from build123d import *

# Parameters (mm, degrees)
F0_R     = 25
F0_R_2   = 1.25
F1_DEPTH = 3


with BuildPart() as f1:
    # F0 (on Top) → F1 (new body)
    with BuildSketch(Plane.XY):
        Circle(F0_R)
        with BuildLine():
            Line((-2, -21.25), (-2, -19.25))
            ThreePointArc((-2, -19.25), (0, -17.25), (2, -19.25))
            Line((2, -19.25), (2, -21.25))
            ThreePointArc((2, -21.25), (0, -23.25), (-2, -21.25))
        make_face(mode=Mode.SUBTRACT)
        with Locations((0, -11.25)):
            Circle(F0_R_2, mode=Mode.SUBTRACT)
        with BuildLine():
            Line((-19.25, -2), (-21.25, -2))
            ThreePointArc((-21.25, -2), (-23.25, 0), (-21.25, 2))
            Line((-21.25, 2), (-19.25, 2))
            ThreePointArc((-19.25, 2), (-17.25, 0), (-19.25, -2))
        make_face(mode=Mode.SUBTRACT)
        with Locations((-11.25, 0)):
            Circle(F0_R_2, mode=Mode.SUBTRACT)
        with Locations((11.25, 0)):
            Circle(F0_R_2, mode=Mode.SUBTRACT)
        with Locations((0, 11.25)):
            Circle(F0_R_2, mode=Mode.SUBTRACT)
        with BuildLine():
            ThreePointArc((21.25, 2), (23.25, 0), (21.25, -2))
            Line((21.25, -2), (19.25, -2))
            ThreePointArc((19.25, -2), (17.25, 0), (19.25, 2))
            Line((19.25, 2), (21.25, 2))
        make_face(mode=Mode.SUBTRACT)
        with BuildLine():
            Line((2, 21.25), (2, 19.25))
            ThreePointArc((2, 19.25), (0, 17.25), (-2, 19.25))
            Line((-2, 19.25), (-2, 21.25))
            ThreePointArc((-2, 21.25), (0, 23.25), (2, 21.25))
        make_face(mode=Mode.SUBTRACT)
    extrude(amount=F1_DEPTH)


solid = f1.part
CAD build for the part. Positions are in the model's coordinates, mm. Round coordinates to 2 decimals unless told otherwise and drop trailing zeros. Write each loop counter-clockwise with the first axis right and the second up, starting at its lowest first coordinate (ties: lowest second). Pieces come first, ordered by that corner, then holes.
(1) Probe line 1 along Y through (x, z) = (0, 2.45); line 2 along X through (y, z) = (-0.5, 2.2) (1 decimal). List the from-to ranges inside material, lowest first.
(2) Mould opens along Y. For faces 1 (the face through (23.846, 7.509, 1.479)), 2 (the face through (0, 0, 0)), 3 (the face through (0.04, -23.25, 1.48)) say: pulls with the +Y half, pulls with the -Y half, needs draft (parallel to the pull), parting line crosses it, or undercut.
(3) Slice it at A-A, the plane x = 20. Write the cut outline in (y, z), and give its area (3 significant figures).
(4) Slice it at B-B, the plane z = 0.5. Count the separate pieces of the cut face and the enclosed holes in it, and give its area (3 significant figures).
(5) Slice it at D-D, the plane y = 11.25. Write the cut outline in (x, z).
(6) Drop flat-ended pins along their axis: P1, Ø1, axis at x = -20.5, z = 1.5, coming from the -Y side; P2, Ø0.6, axis at y = 20.5, z = 1, coming from the -X side; P3, Ø4, axis at x = 11.25, y = 0, coming from the -Z side; P4, Ø1, axis at y = 20, z = 2, coming from the +X side. Give the stop position or say it passes through.
(7) Slice it at C-C, the plane x = 0. Write the cut outline in (y, z), and give its area (3 significant figures).
From the geometry:
1. line 1: y = -25 to -23.25, -17.25 to -12.5, -10 to 10, 12.5 to 17.25, 23.25 to 25
1. line 2: x = -25 to -23.2, -17.3 to -12.4, -10.1 to 10.1, 12.4 to 17.3, 23.2 to 25
2. face 1: parting line crosses it
2. face 2: needs draft
2. face 3: undercut
3. outline: (-15, 0) - (-2, 0) - (-2, 3) - (-15, 3) - close; (2, 0) - (15, 0) - (15, 3) - (2, 3) - close
3. area: 78.0 mm2
4. separate pieces: 1
4. enclosed holes: 8
4. area: 1,860 mm2
5. outline: (-22.33, 0) - (-1.25, 0) - (-1.25, 3) - (-22.33, 3) - close; (1.25, 0) - (22.33, 0) - (22.33, 3) - (1.25, 3) - close
6. P1: stops at y = -15
6. P2: stops at x = -14.73
6. P3: stops at z = 0
6. P4: stops at x = 15.64
7. outline: (-25, 0) - (-23.25, 0) - (-23.25, 3) - (-25, 3) - close; (-17.25, 0) - (-12.5, 0) - (-12.5, 3) - (-17.25, 3) - close; (-10, 0) - (10, 0) - (10, 3) - (-10, 3) - close; (12.5, 0) - (17.25, 0) - (17.25, 3) - (12.5, 3) - close; (23.25, 0) - (25, 0) - (25, 3) - (23.25, 3) - close
7. area: 99.0 mm2
